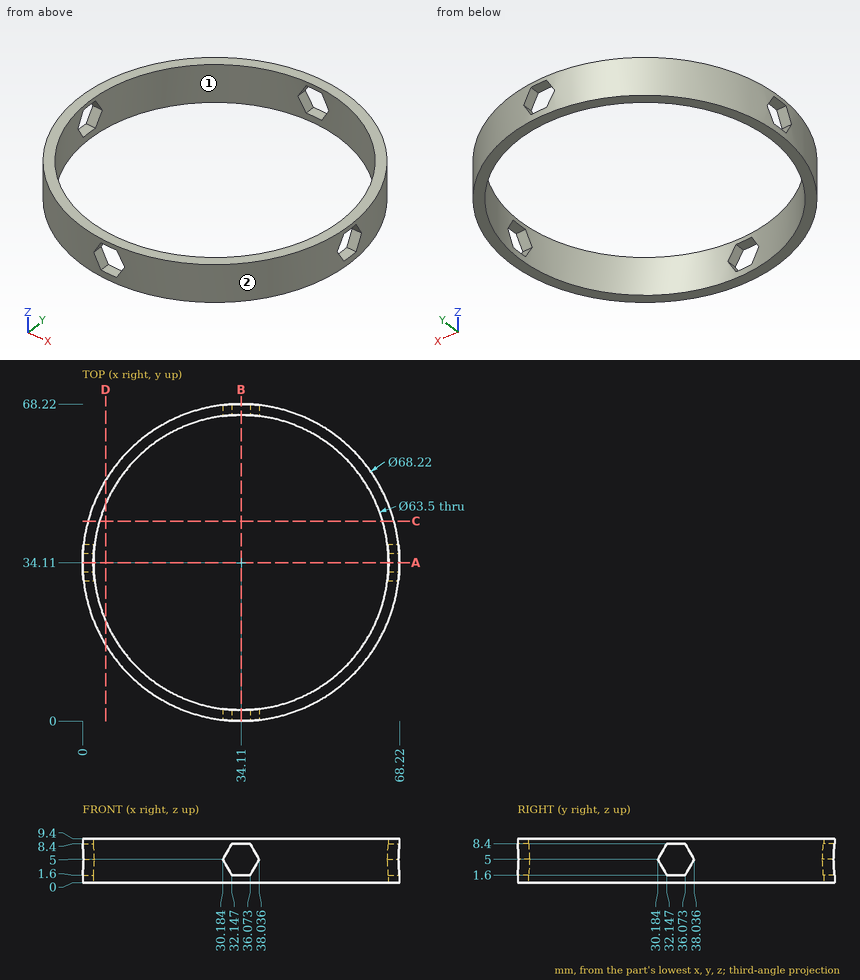
Verification items for this drawing (mm, ordinates from the low corner). Coordinates: 2 decimals unless noted, no trailing zeros. Loops run counter-clockwise (first coordinate to the right, second up) from the corner with the lowest first, then second, coordinate; pieces in that order, holes last.
Item 1: Sectioned sample at C-C, the plane y = 43. Record the boundary of the cut face in (x, z), then the cut area to 3 significant figures.
Item 2: Thickness scan on line 1 (X direction, y = 63, z = 6.5); line 2 (X direction, y = 17, z = 2.5); line 3 (Y direction, x = 15, z = 4.75). Record the ranges inside material, lowest first.
Item 3: Sectioned sample at D-D, the plane x = 5. Record the boundary of the cut face in (y, z), then the cut area to 4 significant figures.
Item 4: Release check for a two-part mould opening along Y. For the marked faces 1 and 2 record: released by +Y, released by -Y, zero draft, split by the parting line, or undercut.
Item 5: Go/stop test with flat-tipped pins: pin 1 Ø0.7 at (x, y) = (67, 35) entering from -Z; pin 2 Ø1.5 at (x, z) = (55, 1.5) entering from -Y; pin 3 Ø2 at (x, z) = (25, 7) entering from -Y; pin 4 Ø1.5 at (x, z) = (55, 7) entering from +Y. Record where each tip stops, or that it passes through.
Item 6: Sectioned sample at A-A, the plane y = 34.11. Record the boundary of the cut face in (x, z).
Check result:
1. outline: (1.18, 0) - (3.63, 0) - (3.63, 9.4) - (1.18, 9.4) - close; (64.59, 0) - (67.04, 0) - (67.04, 9.4) - (64.59, 9.4) - close
1. area: 46.1 mm2
2. line 1: x = 15.98 to 20.94, 47.28 to 52.24
2. line 2: x = 4.6 to 7.36, 60.86 to 63.62
2. line 3: y = 5.86 to 8.76, 59.46 to 62.36
3. outline: (16.33, 0) - (21.43, 0) - (21.43, 9.4) - (16.33, 9.4) - close; (46.79, 0) - (51.89, 0) - (51.89, 9.4) - (46.79, 9.4) - close
3. area: 95.95 mm2
4. face 1: undercut
4. face 2: split by the parting line
5. pin 1: stops at z = 0
5. pin 2: stops at y = 6.58
5. pin 3: stops at y = 0.98
5. pin 4: stops at y = 61.64
6. outline: (0, 0) - (2.36, 0) - (2.36, 1.6) - (0, 1.6) - close; (0, 8.4) - (2.36, 8.4) - (2.36, 9.4) - (0, 9.4) - close; (65.86, 0) - (68.22, 0) - (68.22, 1.6) - (65.86, 1.6) - close; (65.86, 8.4) - (68.22, 8.4) - (68.22, 9.4) - (65.86, 9.4) - close
